```python
from build123d import *

# Parameters (mm, degrees)
EXTRUDE_1_DEPTH     = 33.1
CUT_EXTRUDE_START   = -5
SKETCH_2_R          = 5
CUT_EXTRUDE_1_DEPTH = 5
SKETCH_3_W          = 1.1
SKETCH_3_H          = 0.8
EXTRUDE_2_DEPTH     = 5


with BuildPart() as part:
    # 草图1 → 凸台-拉伸1 (new body)
    with BuildSketch(Plane.XY):
        with BuildLine():
            Line((-3.9, -5.2), (3.9, -5.2))
            ThreePointArc((3.9, -5.2), (0, 6.5), (-3.9, -5.2))
        make_face()
    extrude(amount=EXTRUDE_1_DEPTH)

    # 草图2 → 切除-拉伸1 (cut)
    with BuildSketch(Plane.XY.offset(33.1).offset(CUT_EXTRUDE_START)):
        with BuildLine():
            Line((-3.9, -5.2), (3.9, -5.2))
            ThreePointArc((3.9, -5.2), (0, 6.5), (-3.9, -5.2))
        make_face()
        Circle(SKETCH_2_R, mode=Mode.SUBTRACT)
    extrude(amount=CUT_EXTRUDE_1_DEPTH, mode=Mode.SUBTRACT)

    # 草图3 → 凸台-拉伸2 (add)
    with BuildSketch(Plane(origin=(0, -5.2, 0), x_dir=(1, 0, 0), z_dir=(0, 0, 1))):
        with Locations((0, 10.2)):
            Rectangle(SKETCH_3_W, SKETCH_3_H)
        with Locations((0, 0.2)):
            Rectangle(SKETCH_3_W, SKETCH_3_H)
    extrude(amount=-EXTRUDE_2_DEPTH)


solid = part.part
```
Check sheet for the modelled part. Datum: model origin and axes. Units: mm. A direction names the side the tool comes from. Coordinates: 2 decimals unless noted, no trailing zeros. Write each loop counter-clockwise with the first axis right and the second up, starting at its lowest first coordinate (ties: lowest second). Pieces come first, ordered by that corner, then holes. Notation, with made-up numbers: M 9,56 L 43,56 A15 ccw 43,77 Z; hole C -30.75,57 d1. An arc over 180 degrees is marked long. Use one line per item in the form item = value.
Item 1: Sectioned sample at B-B, the plane y = 0.5. Record the cut outline in (x, z), and give its area (3 significant figures).
Answer below:
outline = M -6.48,0 L 6.48,0 L 6.48,28.1 L 4.97,28.1 L 4.97,33.1 L -4.97,33.1 L -4.97,28.1 L -6.48,28.1 Z
area = 414 mm^2
Item 2: Sectioned sample at D-D, the plane x = 0. Record the cut outline in (y, z).
Answer below:
outline = M -5.4,-5 L -4.6,-5 L -4.6,0 L 4.6,0 L 4.6,-5 L 5.4,-5 L 5.4,0 L 6.5,0 L 6.5,28.1 L 5,28.1 L 5,33.1 L -5,33.1 L -5,28.1 L -5.2,28.1 L -5.2,0 L -5.4,0 Z
Item 3: Sectioned sample at C-C, the plane z = 19. Record the cut outline in (x, y).
Answer below:
outline = M -3.9,-5.2 L 3.9,-5.2 A6.5 ccw long Z
Item 4: Gauge pin test, flat ends, axial feed: pin 1 Ø1.2 at (x, z) = (0, -3) entering from +Y; pin 2 Ø4 at (y, z) = (3.5, 19.5) entering from +X; pin 3 Ø0.6 at (y, z) = (-5, -3.5) entering from -X. Record the tip position at first contact, or that the pin passes through.
Answer below:
pin_1 = 5.4
pin_2 = 6.32
pin_3 = -0.55
Item 5: Material ranges on L1, parallel to Z at x = 3.5, y = 5; L2, parallel to Z at x = 0, y = -2.75; L3, parallel to Y at x = 0.25, z = 19, recorded low to high. Write a range as from..to.
Answer below:
L1 = 0..28.1
L2 = 0..33.1
L3 = -5.2..6.5
Item 6: Release check for a two-part mould opening along Y. For faces 4 (the face through (-1.08, -4.88, 30.56)), 5 (the face through (0, 4.6, -2)), 6 (the face through (0, -4.6, -2)), 7 (the face through (0, 5, -5)) record: pulls with the +Y half, pulls with the -Y half, needs draft (parallel to the pull), parting line crosses it, or undercut.
Answer below:
face_4 = parting line crosses it
face_5 = undercut
face_6 = undercut
face_7 = needs draft
Item 7: Set-up check for faces 1 (the face through (-0.55, 5, -2)), 2 (the face through (0.55, 5, -2)), 3 (the face through (-2, 5, 28.1)): record each of +Z, -Z, +X, -X, +Y, -Y from which the full face is reachable in a straight line by a thin tool's end or side.
Answer below:
face_1 = -Z, -X, +Y, -Y
face_2 = -Z, +X, +Y, -Y
face_3 = +Z
Item 8: Sectioned sample at A-A, the plane x = 2.75. Record the cut outline in (y, z), and give its area (3 significant figures).
Answer below:
outline = M -5.2,0 L 5.89,0 L 5.89,28.1 L 4.18,28.1 L 4.18,33.1 L -4.18,33.1 L -4.18,28.1 L -5.2,28.1 Z
area = 353 mm^2
